from build123d import *

# Parameters (mm, degrees)
F0_R     = 15.875
F0_R_2   = 12.7
F1_DEPTH = 15.875
F0_R_3   = 19.05
F2_DEPTH = 3.175
F4_DEPTH = 15.876


with BuildPart() as f1:
    # F0 (on Front) → F1 (new body)
    with BuildSketch(Plane.XZ):
        Circle(F0_R)
        Circle(F0_R_2, mode=Mode.SUBTRACT)
    extrude(amount=F1_DEPTH)

    # F0 (on Front) → F2 (join)
    with BuildSketch(Plane.XZ):
        Circle(F0_R_3)
        Circle(F0_R, mode=Mode.SUBTRACT)
    extrude(amount=F2_DEPTH)

    # F3 (on face) → F4 (cut, through all)
    with BuildSketch(Plane(origin=(0, 0, 0), x_dir=(-1, 0, 0), z_dir=(0, 1, 0))):
        with BuildLine():
            Line((19.03372, 0.7874), (12.675567, 0.7874))
            ThreePointArc((12.675567, 0.7874), (12.69389, 0.393889), (12.7, 0))
            ThreePointArc((12.7, 0), (12.69389, -0.393889), (12.675567, -0.7874))
            Line((12.675567, -0.7874), (19.03372, -0.7874))
            ThreePointArc((19.03372, -0.7874), (19.04593, -0.393784), (19.05, 0))
            ThreePointArc((19.05, 0), (19.04593, 0.393784), (19.03372, 0.7874))
        make_face()
    extrude(amount=-F4_DEPTH, mode=Mode.SUBTRACT)


solid = f1.part
The model under review builds one solid part; all positions refer to its coordinate system, in mm. A direction names the side the tool comes from. Round coordinates to 2 decimals unless told otherwise and drop trailing zeros. Loops run counter-clockwise (first coordinate to the right, second up) from the corner with the lowest first, then second, coordinate; pieces in that order, holes last. Notation, with made-up numbers: M 37,-33 L 96,-33 A22 cw 96,-21 Z; hole C 80,72 d6. An arc over 180 degrees is marked long. Answer as CSV lines item,"result". Start each with the question number.
Item 1: Consider section D-D (z = 14.5). Write out the cut boundary in (x, y) (3 decimals), then the cut area to 3 significant figures.
Item 2: Wall thickness on line 1 (Y direction, x = 1, z = 16.5) (3 decimals); line 2 (Z direction, x = 8, y = -12); line 3 (Z direction, x = 11.5, y = -11.25): over which ranges is each line inside the solid? List them lowest first. Write a range as [from, to].
Item 3: Mouldability with a two-part tool opening along Z and no side actions: class faces 1 (the face through (12.4, 0, -4)), 2 (the face through (-14, -6, 0.787)) as released by +Z, released by -Z, zero draft, split by the parting line, or undercut.
Item 4: Consider section A-A (x = 0). Write out the cut boundary in (y, z) (3 decimals).
Item 5: Consider section C-C (x = 15). Write out the cut boundary in (y, z) (3 decimals).
Item 6: Consider section B-B (z = 10). Write out the cut boundary in (x, y) (3 decimals), then the cut area to 3 significant figures.
Item 7: Insertion check: P1, Ø8, axis at y = -13, z = 15, coming from the -X side; P2, Ø5, axis at x = -9.5, y = -13, coming from the -Z side; P3, Ø4, axis at y = -9, z = -3, coming from the -X side. Each pin has a flat end and moves straight along its axis. Give the tip position at first contact, or say it passes through.
Item 8: For faces 3 (the face through (-4, -3.175, 16)), 4 (the face through (11, -15.875, 7)), 5 (the face through (-15, -6, -0.787)), list the 3-axis set-ups (+Z, -Z, +X, -X, +Y, -Y) from which the entire face can be reached by the end or side of a thin tool; tool diameter is ignored.
Answer:
1,outline,"M -12.355,-3.175 L -6.463,-3.175 L -6.463,-15.875 L 6.463,-15.875 L 6.463,-3.175 L 12.355,-3.175 L 12.355,0 L -12.355,0 Z"
1,area,"243 mm^2"
2,line 1,"y = [-3.175, 0]"
2,line 2,"z = [-13.71, -9.86], [9.86, 13.71]"
2,line 3,"z = [-10.94, -5.39], [5.39, 10.94]"
3,face 1,"zero draft"
3,face 2,"undercut"
4,outline,"M -15.875,-15.875 L -3.175,-15.875 L -3.175,-19.05 L 0,-19.05 L 0,-12.7 L -15.875,-12.7 Z; M -15.875,12.7 L 0,12.7 L 0,19.05 L -3.175,19.05 L -3.175,15.875 L -15.875,15.875 Z"
5,outline,"M -15.875,-5.198 L -3.175,-5.198 L -3.175,-11.743 L 0,-11.743 L 0,11.743 L -3.175,11.743 L -3.175,5.198 L -15.875,5.198 Z"
6,outline,"M -16.214,-3.175 L -12.329,-3.175 L -12.329,-15.875 L -7.829,-15.875 L -7.829,0 L -16.214,0 Z; M 7.829,-15.875 L 12.329,-15.875 L 12.329,-3.175 L 16.214,-3.175 L 16.214,0 L 7.829,0 Z"
6,area,"168 mm^2"
7,P1,"stops at x = -11.45"
7,P2,"stops at z = -14.25"
7,P3,"stops at x = -15.84"
8,face 3,"-Y"
8,face 4,"+Z, -Z, +X, -X, -Y"
8,face 5,"-X, +Y, -Y"
